```python
from build123d import *

# Parameters (mm, degrees)
CYLINDER003_R     = 2
CYLINDER003_DEPTH = 10
CYLINDER004_R     = 2
CYLINDER004_DEPTH = 30
CYLINDER001_R     = 10.2
CYLINDER001_DEPTH = 10
BOX_W             = 10
BOX_H             = 15
BOX_DEPTH         = 10
CYLINDER_R        = 15
CYLINDER_DEPTH    = 10


with BuildPart() as cylinder003:
    # Cylinder003 → Cylinder003 (new body)
    with BuildSketch(Plane(origin=(10, 20, 0), x_dir=(0, 0, 1), z_dir=(-1, 0, 0))):
        Circle(CYLINDER003_R)
    extrude(amount=CYLINDER003_DEPTH)


with BuildPart() as cylinder004:
    # Cylinder004 → Cylinder004 (new body)
    with BuildSketch(Plane.ZY.offset(-15)):
        Circle(CYLINDER004_R)
    extrude(amount=CYLINDER004_DEPTH)


with BuildPart() as negative_fusion:
    # Cylinder001 → Cylinder001 (new body)
    with BuildSketch(Plane.XY.offset(-5)):
        Circle(CYLINDER001_R)
    extrude(amount=CYLINDER001_DEPTH)

    # Fusion: union Cylinder003, Cylinder004
    add(cylinder003.part)
    add(cylinder004.part)


with BuildPart() as cube:
    # Box → Box (new body)
    with BuildSketch(Plane(origin=(0, 10, -5), x_dir=(1, 0, 0), z_dir=(0, 0, 1))):
        with Locations((5, 7.5)):
            Rectangle(BOX_W, BOX_H)
    extrude(amount=BOX_DEPTH)


with BuildPart() as cut:
    # Cylinder → Cylinder (new body)
    with BuildSketch(Plane.XY.offset(-5)):
        Circle(CYLINDER_R)
    extrude(amount=CYLINDER_DEPTH)

    # Fusion001: union Cube
    add(cube.part)

    # Cut: cut Negative Fusion
    add(negative_fusion.part, mode=Mode.SUBTRACT)


solid = cut.part
```
Design review of the part built by this model. Coordinates are the model's own, in mm. A direction names the side the tool comes from. Give positions to 0.01 mm unless a question says otherwise; leave off trailing zeros. Loops run counter-clockwise (first coordinate to the right, second up) from the corner with the lowest first, then second, coordinate; pieces in that order, holes last. Notation, with made-up numbers: (29, 73.25) -> (34, 73.25) arc R5 cw to (34, 78.25) -> close; hole circle Ø4 at (65.25, 22.5). An arc over 180 degrees is marked (long way). Write each question's results on one line, items separated by ' | '.
Q1. For pin 1 Ø5 at (y, z) = (21.5, 0.5) entering from -X; pin 2 Ø2 at (y, z) = (13, -4) entering from -X; pin 3 Ø4 at (y, z) = (14.5, 3) entering from -X, all flat-tipped, find the tip position at first contact; note any pin that passes through.
Reply:
pin 1: stops at x = 0 | pin 2: stops at x = -9 | pin 3: stops at x = -8.29
Q2. Take a section at B-B, the plane y = -1.5. Write out the cut boundary in (x, z).
Reply:
outline: (-14.92, -5) -> (-10.09, -5) -> (-10.09, -1.32) -> (-14.92, -1.32) -> close; (-14.92, 1.32) -> (-10.09, 1.32) -> (-10.09, 5) -> (-14.92, 5) -> close; (10.09, -5) -> (14.92, -5) -> (14.92, -1.32) -> (10.09, -1.32) -> close; (10.09, 1.32) -> (14.92, 1.32) -> (14.92, 5) -> (10.09, 5) -> close
Q3. Take a section at D-D, the plane x = -2. Write out the cut boundary in (y, z).
Reply:
outline: (-14.87, -5) -> (-10, -5) -> (-10, 5) -> (-14.87, 5) -> close; (10, -5) -> (14.87, -5) -> (14.87, 5) -> (10, 5) -> close
Q4. Take a section at A-A, the plane x = 5.5. Write out the cut boundary in (y, z).
Reply:
outline: (-13.96, -5) -> (-8.59, -5) -> (-8.59, 5) -> (-13.96, 5) -> close; (8.59, -5) -> (25, -5) -> (25, 5) -> (8.59, 5) -> close; hole circle Ø4 at (20, 0)
Q5. Take a section at C-C, the plane z = 1. Write out the cut boundary in (x, y).
Reply:
outline: (-14.9, -1.73) arc R15 ccw to (14.9, -1.73) -> (10.05, -1.73) arc R10.2 cw to (-10.05, -1.73) -> close; (-14.9, 1.73) -> (-10.05, 1.73) arc R10.2 cw to (10.05, 1.73) -> (14.9, 1.73) arc R15 ccw to (10, 11.18) -> (10, 18.27) -> (0, 18.27) -> (0, 15) arc R15 ccw to start; (0, 21.73) -> (10, 21.73) -> (10, 25) -> (0, 25) -> close
Q6. Machinability: for faces 5 (the face through (5, 22, 0)), 6 (the face through (10, 18, 1)), which of the approach directions +Z, -Z, +X, -X, +Y, -Y give a long, thin tool a straight path to every point of the face, cutting with its end or side? Answer none if there is none.
Reply:
face 5: +X, -X | face 6: +Z, -Z, +X, +Y
Q7. The part is to be moulded in two halves that separate along Y. For faces 1 (the face through (12.536, -1.774, 0.923)), 2 (the face through (0, 17.7, -0.1)), 3 (the face through (-12.466, -1.774, 0.923)), 4 (the face through (5, 25, 0)), say which applies: +Y half, -Y half, draft (parallel to the pull), parting line (faces both ways), or undercut.
Reply:
face 1: undercut | face 2: draft | face 3: undercut | face 4: +Y half
Q8. Wall thickness on L1, parallel to Y at x = 2.5, z = 0; L2, parallel to Z at x = 11, y = 0; L3, parallel to Y at x = 4, z = 4.5: over which ranges is each line inside the solid? List them lowest first.
Reply:
L1: y = -14.79 to -9.89, 9.89 to 18, 22 to 25 | L2: z = -5 to -2, 2 to 5 | L3: y = -14.46 to -9.38, 9.38 to 25
